The listing builds one solid part. Answer for the finished solid, in the listing's coordinates (mm). Face numbers are marked on the shaded views. A direction names the side the tool comes from. Round coordinates to 2 decimals unless told otherwise and drop trailing zeros. Write each loop counter-clockwise with the first axis right and the second up, starting at its lowest first coordinate (ties: lowest second). Pieces come first, ordered by that corner, then holes. Notation, with made-up numbers: M 24.5,-24 L 37.5,-24 A16 cw 37.5,-2 Z; hole C -17.5,14.25 d1. An arc over 180 degrees is marked long. Put each result on its own line as item: value. Start each with the question number.
```python
from build123d import *

# Parameters (mm, degrees)
SKETCH_1_R          = 7.75
EXTRUDE_1_DEPTH     = 24
EXTRUDE_START       = -24
EXTRUDE_2_DEPTH     = 24
SKETCH_3_W          = 50
SKETCH_3_H          = 3.75
EXTRUDE_3_DEPTH     = 24
SKETCH_4_W          = 80
SKETCH_4_H          = 6
CUT_EXTRUDE_1_DEPTH = 24
FILLET_1_R          = 2
SKETCH_5_W          = 7.752834923
SKETCH_5_H          = 5
CUT_EXTRUDE_2_DEPTH = 24
SKETCH_6_R          = 1.75
CUT_EXTRUDE_3_DEPTH = 24
SKETCH_7_R          = 1.75
CUT_EXTRUDE_4_DEPTH = 3
SKETCH_8_W          = 10.83484861
SKETCH_8_H          = 3
CUT_EXTRUDE_5_DEPTH = 75.375029438
SKETCH_9_R          = 1.75
CUT_EXTRUDE_6_DEPTH = 3
SKETCH_10_R         = 3
CUT_EXTRUDE_7_DEPTH = 4


with BuildPart() as part:
    # 草图1 → 凸台-拉伸1 (new body)
    with BuildSketch(Plane(origin=(0, 0, 0), x_dir=(1, 0, 0), z_dir=(0, 1, 0))):
        with BuildLine():
            Line((-50.83484861, -4), (50.83484861, -4))
            ThreePointArc((50.83484861, -4), (65.477225575, 8.366600265), (60, -10))
            Line((60, -10), (-60, -10))
            ThreePointArc((-60, -10), (-65.477225575, 8.366600265), (-50.83484861, -4))
        make_face()
        with Locations(Location((-60, 0, 0), (0, 0, 270))):
            Circle(SKETCH_1_R, mode=Mode.SUBTRACT)
        with Locations(Location((60, 0, 0), (0, 0, 270))):
            Circle(SKETCH_1_R, mode=Mode.SUBTRACT)
    extrude(amount=EXTRUDE_1_DEPTH)

    # 草图2 → 凸台-拉伸2 (add)
    with BuildSketch(Plane(origin=(0, 24, 0), x_dir=(1, 0, 0), z_dir=(0, 1, 0)).offset(EXTRUDE_START)):
        with BuildLine():
            ThreePointArc((-60, 10), (-52.928932188, 7.071067812), (-50, 0))
            Line((-50, 0), (50, 0))
            ThreePointArc((50, 0), (52.928932188, 7.071067812), (60, 10))
            Line((60, 10), (-60, 10))
        make_face()
    extrude(amount=EXTRUDE_2_DEPTH)

    # 草图3 → 凸台-拉伸3 (add)
    with BuildSketch(Plane.XZ):
        with Locations((0, 1.875)):
            Rectangle(SKETCH_3_W, SKETCH_3_H)
    extrude(amount=-EXTRUDE_3_DEPTH)

    # 草图4 → 切除-拉伸1 (cut)
    with BuildSketch(Plane.XZ):
        with Locations((0, 7)):
            Rectangle(SKETCH_4_W, SKETCH_4_H)
        with Locations((0, -7)):
            Rectangle(SKETCH_4_W, SKETCH_4_H)
    extrude(amount=-CUT_EXTRUDE_1_DEPTH, mode=Mode.SUBTRACT)

    # 圆角1
    fillet_1_edges = [part.edges().sort_by_distance(p)[0] for p in [
        (40, 12, -10),
        (-40, 12, -10),
    ]]
    fillet(fillet_1_edges, radius=FILLET_1_R)

    # 草图5 → 切除-拉伸2 (cut)
    with BuildSketch(Plane.XZ):
        with Locations((68.12542242, 0)):
            Rectangle(SKETCH_5_W, SKETCH_5_H)
        with Locations((-68.12542242, 0)):
            Rectangle(SKETCH_5_W, SKETCH_5_H)
    extrude(amount=-CUT_EXTRUDE_2_DEPTH, mode=Mode.SUBTRACT)

    # 草图6 → 切除-拉伸3 (cut)
    with BuildSketch(Plane(origin=(0, 0, -4), x_dir=(-1, 0, 0), z_dir=(0, 0, -1))):
        with Locations((-6, 12)):
            Circle(SKETCH_6_R)
        with Locations((6, 12)):
            Circle(SKETCH_6_R)
    extrude(amount=-CUT_EXTRUDE_3_DEPTH, mode=Mode.SUBTRACT)

    # 草图7 → 切除-拉伸4 (cut)
    with BuildSketch(Plane.XY.offset(10)):
        with Locations((45, 7)):
            Circle(SKETCH_7_R)
        with Locations((45, 17)):
            Circle(SKETCH_7_R)
    extrude(amount=-CUT_EXTRUDE_4_DEPTH, mode=Mode.SUBTRACT)

    # 草图8 → 切除-拉伸5 (cut, through all)
    with BuildSketch(Plane.XZ):
        with Locations((45.417424305, 5.5)):
            Rectangle(SKETCH_8_W, SKETCH_8_H)
        with Locations((-45.417424305, 5.5)):
            Rectangle(SKETCH_8_W, SKETCH_8_H)
    extrude(amount=-CUT_EXTRUDE_5_DEPTH, mode=Mode.SUBTRACT)

    # 草图9 → 切除-拉伸6 (cut)
    with BuildSketch(Plane.XY.offset(10)):
        with Locations((-45, 7)):
            Circle(SKETCH_9_R)
        with Locations((-45, 17)):
            Circle(SKETCH_9_R)
    extrude(amount=-CUT_EXTRUDE_6_DEPTH, mode=Mode.SUBTRACT)

    # 草图10 → 切除-拉伸7 (cut)
    with BuildSketch(Plane(origin=(0, 0, -4), x_dir=(-1, 0, 0), z_dir=(0, 0, -1))):
        with Locations((6, 12)):
            Circle(SKETCH_10_R)
        with Locations((-6, 12)):
            Circle(SKETCH_10_R)
    extrude(amount=-CUT_EXTRUDE_7_DEPTH, mode=Mode.SUBTRACT)


solid = part.part
```
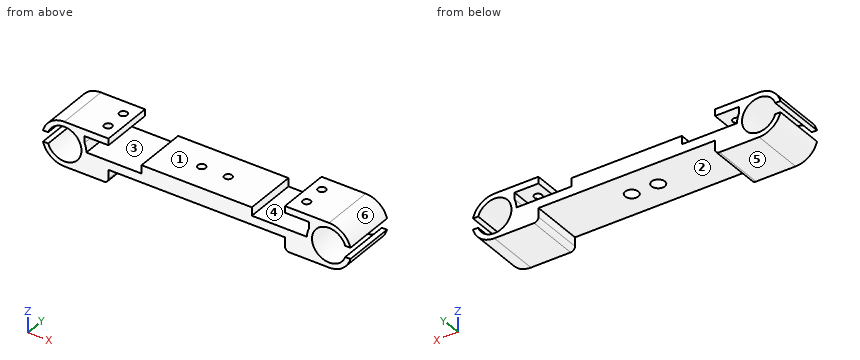
Item 1: Determine the mould class of the marked faces 4, 5 and 6 for opening direction X: released by +X, released by -X, zero draft, split by the parting line, or undercut.
Item 2: Section A-A (x = -6) is taken. Give the vertices of the cut face in (y, z), and give its area (3 significant figures).
Item 3: Which of the six approach directions +Z, -Z, +X, -X, +Y, -Y give full straight-line access (tool end or side, diameter ignored) to the marked faces 1, 2 and 3?
Item 4: Section D-D (y = 12) is taken. Count the separate pieces of the cut face and the enclosed holes in it, and give its area (3 significant figures).
Item 5: Flat-ended cylindrical pins translate along their axes: pin 1 (2.5 mm diameter, centred on x = 68, y = 12.5, fed in from +Z); pin 2 (3 mm diameter, centred on x = -45, y = 17, fed in from +Z); pin 3 (4.5 mm diameter, centred on y = 17.5, z = -6, fed in from -X); pin 4 (2 mm diameter, centred on x = -6, y = 12, fed in from +Z). Find the tip coordinate at first contact, or state that the pin passes through.
Item 6: Consider line 1 along Y through (x, z) = (-45, 8.8); line 2 along X through (y, z) = (1.5, 0.25); line 3 along X through (y, z) = (1.5, -4.25). Determine where each line is inside the solid, lowest interval first. Write a range as [from, to].
Item 7: Section C-C (z = 5.25) is taken. Give the vertices of the cut face in (x, y).
Output values:
1. face 4: undercut
1. face 5: zero draft
1. face 6: released by +X
2. outline: M 0,-4 L 9,-4 L 9,0 L 10.25,0 L 10.25,3.75 L 0,3.75 Z; M 13.75,0 L 15,0 L 15,-4 L 24,-4 L 24,3.75 L 13.75,3.75 Z
2. area: 149 mm^2
3. face 1: +Z, +Y, -Y
3. face 2: -Z, +Y, -Y
3. face 3: +Y, -Y
4. separate pieces: 3
4. enclosed holes: 0
4. area: 998 mm^2
5. pin 1: stops at z = 7.38
5. pin 2: stops at z = 0
5. pin 3: stops at x = -69.27
5. pin 4: passes through
6. line 1: y = [0, 5.25], [8.75, 15.25], [18.75, 24]
6. line 2: x = [-52.25, -50], [-25, 25], [50, 52.25]
6. line 3: x = [-69.05, -66.48], [-53.52, -40], [40, 53.52], [66.48, 69.05]
7. outline: M -68.51,0 L -65.7,0 L -65.7,24 L -68.51,24 Z; M -54.3,0 L -50.83,0 L -50.83,24 L -54.3,24 Z; M 50.83,0 L 54.3,0 L 54.3,24 L 50.83,24 Z; M 65.7,0 L 68.51,0 L 68.51,24 L 65.7,24 Z
